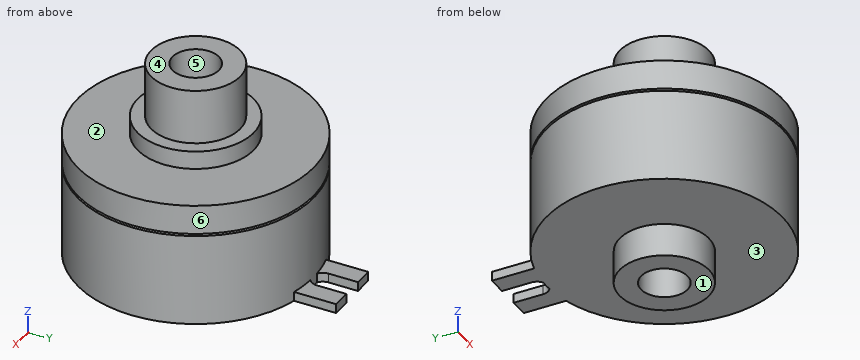
from build123d import *

# Parameters (mm, degrees)
SKETCH1_R           = 9.61
BOSS_EXTRUDE1_DEPTH = 7.087
SKETCH2_R           = 25.4
BOSS_EXTRUDE2_DEPTH = 26.67
SKETCH3_R           = 12.5
BOSS_EXTRUDE3_DEPTH = 3.911
SKETCH4_R           = 9.601
BOSS_EXTRUDE4_DEPTH = 11.811
BOSS_EXTRUDE5_DEPTH = 2
SKETCH5_R           = 5
CUT_EXTRUDE1_DEPTH  = 66.007618523
SKETCH7_OUTSIDE_W   = 71.256
SKETCH7_OUTSIDE_H   = 79.511
SKETCH7_OUTSIDE_R   = 18.771401146
CUT_EXTRUDE2_DEPTH  = 0.5


with BuildPart() as part:
    # Sketch1 → Boss-Extrude1 (new body)
    with BuildSketch(Plane.XY):
        with Locations(Location((0, 0, 0), (0, 0, 180))):
            Circle(SKETCH1_R)
    extrude(amount=BOSS_EXTRUDE1_DEPTH)

    # Sketch2 → Boss-Extrude2 (add)
    with BuildSketch(Plane.XY.offset(7.087)):
        Circle(SKETCH2_R)
    extrude(amount=BOSS_EXTRUDE2_DEPTH)

    # Sketch3 → Boss-Extrude3 (add)
    with BuildSketch(Plane.XY.offset(33.757)):
        Circle(SKETCH3_R)
    extrude(amount=BOSS_EXTRUDE3_DEPTH)

    # Sketch4 → Boss-Extrude4 (add)
    with BuildSketch(Plane.XY.offset(37.668)):
        Circle(SKETCH4_R)
    extrude(amount=BOSS_EXTRUDE4_DEPTH)

    # Sketch6 → Boss-Extrude5 (add)
    with BuildSketch(Plane(origin=(0, 0, 7.087), x_dir=(-1, 0, 0), z_dir=(0, 0, -1))):
        with BuildLine():
            Line((-6.4135, 33.655), (-2.337, 33.655))
            Line((-2.337, 33.655), (-2.337, 27.34))
            ThreePointArc((-2.337, 27.34), (0, 25.003), (2.337, 27.34))
            Line((2.337, 27.34), (2.337, 33.655))
            Line((2.337, 33.655), (6.4135, 33.655))
            Line((6.4135, 33.655), (6.4135, 24.576961117))
            ThreePointArc((6.4135, 24.576961117), (0, -25.4), (-6.4135, 24.576961117))
            Line((-6.4135, 24.576961117), (-6.4135, 33.655))
        make_face()
    extrude(amount=-BOSS_EXTRUDE5_DEPTH)

    # Sketch5 → Cut-Extrude1 (cut, through all)
    with BuildSketch(Plane.XY.offset(49.479)):
        Circle(SKETCH5_R)
    extrude(amount=-CUT_EXTRUDE1_DEPTH, mode=Mode.SUBTRACT)

    # Sketch7 outside → Cut-Extrude2 (cut)
    with BuildSketch(Plane(origin=(0, 0, 26.927), x_dir=(-1, 0, 0), z_dir=(0, 0, -1))):
        with Locations((0, 4.1275)):
            Rectangle(SKETCH7_OUTSIDE_W, SKETCH7_OUTSIDE_H)
        Circle(SKETCH7_OUTSIDE_R, mode=Mode.SUBTRACT)
    extrude(amount=-CUT_EXTRUDE2_DEPTH, mode=Mode.SUBTRACT)


solid = part.part
Read the model definition and answer for the solid it produces. Units are mm, in the model's axes. Face numbers are marked on the shaded views. A direction names the side the tool comes from. Round coordinates to 2 decimals unless told otherwise and drop trailing zeros. Order: outer loops, then holes, each group sorted by start corner. A loop starts at its lowest first (then second) coordinate and runs counter-clockwise, first axis right, second up.
1) For the marked faces 1, 2 and 3, determine the directions among +Z, -Z, +X, -X, +Y, -Y from which every point of the face is accessible in a straight line to the end or side of a thin tool.
2) The part is cut by section C-C on x = 11. Write down the section's boundary in (y, z), plus the area to 3 significant figures.
3) Straight lines are drawn through the part: L1, parallel to Y at x = 0, z = 18; L2, parallel to Z at x = -21.5, y = -7; L3, parallel to X at y = -4.5, z = 16.5. For each, find the intervals that lie inside material, in ascending order.
4) The mould has two halves that part along X. Classify the marked faces 4, 5 and 6: released by +X, released by -X, zero draft, split by the parting line, or undercut.
5) The part is cut by section A-A on x = 0. Write down the section's boundary in (y, z).
6) The part is cut by section D-D on z = 43. Write down the section's boundary in (x, y).
7) Flat-ended cylindrical pins translate along their axes: pin 1 (15 mm diameter, centred on x = 0, y = -7, fed in from -Z); pin 2 (2 mm diameter, centred on y = -13, z = 25.5, fed in from +X); pin 3 (5.5 mm diameter, centred on x = -5, y = 28.5, fed in from +Z); pin 4 (2 mm diameter, centred on y = 29.5, z = 8, fed in from +X). Find the tip coordinate at first contact, or state that the pin passes through.
Resolved:
1. face 1: -Z, +X, -X, +Y, -Y
1. face 2: +Z
1. face 3: -Z
2. outline: (-22.89, 7.09) - (22.89, 7.09) - (22.89, 26.93) - (15.21, 26.93) - (15.21, 27.43) - (22.89, 27.43) - (22.89, 33.76) - (5.94, 33.76) - (5.94, 37.67) - (-5.94, 37.67) - (-5.94, 33.76) - (-22.89, 33.76) - (-22.89, 27.43) - (-15.21, 27.43) - (-15.21, 26.93) - (-22.89, 26.93) - close
2. area: 1,260 mm2
3. L1: y = -25.4 to -5, 5 to 25.4
3. L2: z = 7.09 to 26.93, 27.43 to 33.76
3. L3: x = -25 to -2.18, 2.18 to 25
4. face 4: zero draft
4. face 5: undercut
4. face 6: split by the parting line
5. outline: (-25.4, 7.09) - (-9.61, 7.09) - (-9.61, 0) - (-5, 0) - (-5, 49.48) - (-9.6, 49.48) - (-9.6, 37.67) - (-12.5, 37.67) - (-12.5, 33.76) - (-25.4, 33.76) - (-25.4, 27.43) - (-18.77, 27.43) - (-18.77, 26.93) - (-25.4, 26.93) - close; (5, 0) - (9.61, 0) - (9.61, 7.09) - (25.4, 7.09) - (25.4, 26.93) - (18.77, 26.93) - (18.77, 27.43) - (25.4, 27.43) - (25.4, 33.76) - (12.5, 33.76) - (12.5, 37.67) - (9.6, 37.67) - (9.6, 49.48) - (5, 49.48) - close
6. outline: circle Ø19.2 at (0, 0); hole circle Ø10 at (0, 0)
7. pin 1: stops at z = 0
7. pin 2: stops at x = 22.39
7. pin 3: stops at z = 9.09
7. pin 4: stops at x = 6.41
